Answer from the drawing. Dimensions are ordinates in mm from the lowest x, y and z of the part. Round coordinates to 2 decimals unless told otherwise and drop trailing zeros. Order: outer loops, then holes, each group sorted by start corner. A loop starts at its lowest first (then second) coordinate and runs counter-clockwise, first axis right, second up.
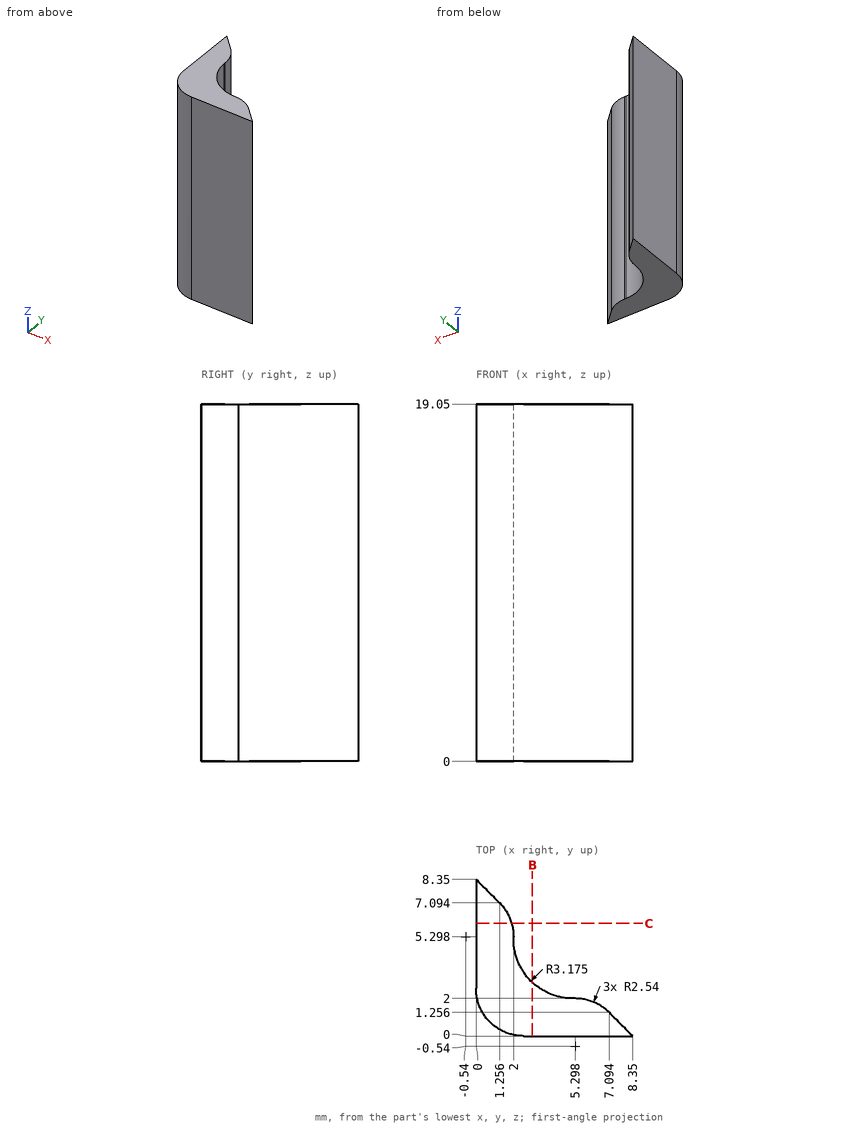
Q1. Straight lines are drawn through the part: probe 1 along Y at (x, z) = (5, 5) (3 decimals); probe 2 along X at (y, z) = (2.25, 17.75); probe 3 along Y at (x, z) = (6.5, 2). For each, find the intervals that lie inside material, in ascending order.
Outcome:
probe 1: y = 0 to 2.005
probe 2: x = 0.02 to 3.94
probe 3: y = 0 to 1.7
Q2. A cutting plane is placed at C-C, the plane y = 6. Give the vertices of the cut face in (x, z), plus the area to 3 significant figures.
Outcome:
outline: (0, 0) - (1.9, 0) - (1.9, 19.05) - (0, 19.05) - close
area: 36.2 mm2
Q3. Flat-ended cylindrical pins translate along their axes: pin 1 (3 mm diameter, centred on y = 2.5, z = 14, fed in from +X); pin 2 (3 mm diameter, centred on x = 5, z = 9.5, fed in from +Y); pin 3 (2 mm diameter, centred on y = 2.5, z = 5.5, fed in from +X). Find the tip coordinate at first contact, or state that the pin passes through.
Outcome:
pin 1: stops at x = 7.35
pin 2: stops at y = 2.48
pin 3: stops at x = 6.81
Q4. A cutting plane is placed at B-B, the plane x = 3. Give the vertices of the cut face in (y, z).
Outcome:
outline: (0, 0) - (2.86, 0) - (2.86, 19.05) - (0, 19.05) - close
